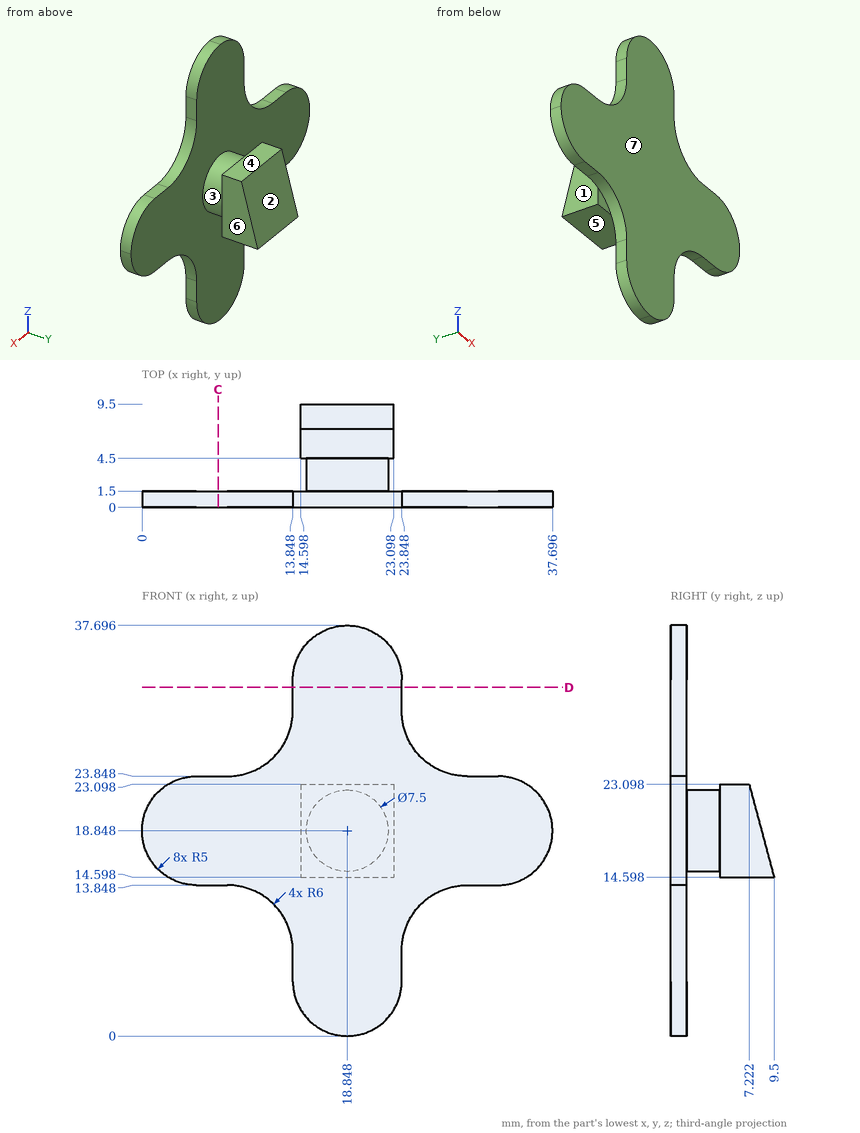
Can you work these out from the drawing? Everything is in mm from the part's minimum corner. A direction names the side the tool comes from. Give positions to 0.01 mm unless a question says otherwise; leave off trailing zeros. Loops run counter-clockwise (first coordinate to the right, second up) from the corner with the lowest first, then second, coordinate; pieces in that order, holes last. Notation, with made-up numbers: (5, 17.25) -> (60, 17.25) arc R27 ccw to (60, 40.25) -> close; hole circle Ø1 at (4.5, 67.5). An arc over 180 degrees is marked (long way). Write item = value, one per line.
1) Suppose I cut it at D-D on z = 32. Write out the boundary of the cut face in (x, y).
Check result:
outline = (13.85, 0) -> (23.85, 0) -> (23.85, 1.5) -> (13.85, 1.5) -> close
2) Will these pins go through, and if not, where does the flat tip stop? pin 1 (4 mm diameter, centred on y = 6, z = 12.5, fed in from +X); pin 2 (5.5 mm diameter, centred on x = 17, y = 7.5, fed in from -Z); pin 3 (1.2 mm diameter, centred on x = 6.5, y = 1, fed in from -Z); pin 4 (2 mm diameter, centred on x = 17, y = 1.5, fed in from +Z).
Check result:
pin_1 = through
pin_2 = 14.6
pin_3 = 13.85
pin_4 = 37.62
3) I need wall thicknesses on L1, parallel to Y at x = 18, z = 24; L2, parallel to Z at x = 19.5, y = 1; L3, parallel to Z at x = 16.5, y = 6. Which ranges of each line are inside material? Lowest first, please. Write a range as from..to.
Check result:
L1 = 0..1.5
L2 = 0.04..37.65
L3 = 14.6..23.1
4) Suppose I cut it at C-C on x = 7. Write out the boundary of the cut face in (y, z), then the cut area to 3 significant figures.
Check result:
outline = (0, 13.85) -> (1.5, 13.85) -> (1.5, 23.85) -> (0, 23.85) -> close
area = 15.0 mm2
5) Thinking about a two-plate mould opening in Y: for the marked faces 1, 2 and 3, which applies, released by +Y, released by -Y, zero draft, split by the parting line, or undercut?
Check result:
face_1 = zero draft
face_2 = released by +Y
face_3 = undercut
6) For the marked faces 4, 5, 6 and 7, which set-ups out of +Z, -Z, +X, -X, +Y, -Y let a thin tool reach every point of the face, with its end or its side?
Check result:
face_4 = +Z, +X, -X, +Y
face_5 = -Z, +X, -X, +Y
face_6 = +Z, -Z, +X, +Y
face_7 = +Z, -Z, +X, -X, -Y
